Solid Edge part; units mm, degrees
sketch "Sketch1" plane through (0, 0, 0) normal (1, 0, 0) x (0, 1, 0)
  circle A0 centre (0, 0) radius 3.5
extrude "Protrusion1" add sketch "Sketch1" along normal mid plane 72
sketch "Sketch2" plane through (0, 0, 0) normal (0, -1, 0) x (1, 0, 0)
  line L0 (-36, 3) -> (-23, 3)
  line L1 (-23, 3) -> (-23, 3.5)
  dimension "D1" = 36
revolve "RevolvedCutout1" cut sketch "Sketch2" angle 360 about axis through (-60, 0, 0) along (1, 0, 0) material side at (-29.5, 0, 3.05)
sketch "Sketch3" plane through (0, 0, 0) normal (0, -1, 0) x (1, 0, 0)
  line L0 (36, 3) -> (2, 3)
  line L1 (2, 3) -> (2, 3.5)
  dimension "D1" = 36
revolve "RevolvedCutout2" cut sketch "Sketch3" angle 360 about axis through (-60, 0, 0) along (1, 0, 0) material side at (19, 0, 3.05)
sketch "Sketch4" plane through (0, 0, 0) normal (0, -1, 0) x (1, 0, 0)
  line L0 (16.5, 2.5) -> (16.5, 3)
  line L1 (21.5, 2.5) -> (16.5, 2.5)
  line L2 (21.5, 2.25) -> (21.5, 2.5)
  line L3 (21.5, 2.25) -> (26, 2.25)
  line L4 (26, 2.25) -> (26, 2)
  line L5 (26, 2) -> (36, 2)
  dimension "D1" = 26
revolve "RevolvedCutout3" cut sketch "Sketch4" angle 360 about axis through (-60, 0, 0) along (1, 0, 0) material side at (16.55, 0, 2.75)
cosmetic_thread "Gewinde_1" thread depth 9.5
fillet "Verrundung_2" radius 0.5 1 edges at (26, 0, -2)
sketch "Sketch5" plane through (0, 0, 0) normal (0, 0, 1) x (1, 0, 0)
  circle A0 centre (-19.75, 0) radius 1.25
extrude "Cutout1" cut sketch "Sketch5" along normal up to next and the other way up to next
sketch "Sketch6" plane through (0, 0, 0) normal (0, 0, 1) x (1, 0, 0)
  circle A0 centre (11.25, 0) radius 1.25
extrude "Cutout2" cut sketch "Sketch6" along normal up to next and the other way up to next
properties material "Stahl - Unlegierter:1.1191 , C45E"
Geometry check sheet. Reference: the model listing, model coordinates, mm. A direction names the side the tool comes from. Round coordinates to 2 decimals unless told otherwise and drop trailing zeros. Order: outer loops, then holes, each group sorted by start corner. A loop starts at its lowest first (then second) coordinate and runs counter-clockwise, first axis right, second up. Notation, with made-up numbers: (43, -23.75) - (76, -23.75) arc R35 ccw to (76, 8.25) - close; hole circle Ø6 at (19, -24.75). An arc over 180 degrees is marked (long way). Use a Markdown table: item, result. Add a question column.
(1) Sectioned sample at B-B, the plane z = 0. Enter the section's corners in (x, y).
(2) Release check for a two-part mould opening along X. For faces 1 (the flat face through (-36, 0, 0)), 2 (the cylindrical face through (-18.595, 0.479, -0.049)), 3 (the cylindrical face through (23.78, -2.23, -0.29)) record: pulls with the +X half, pulls with the -X half, needs draft (parallel to the pull), parting line crosses it, or undercut.
(3) Tool access check on faces 4 (the cylindrical face through (-10.675, 3.233, 1.341)), 5 (the flat face through (2, -1, 3)), 6 (the flat face through (-23, -1, 3)). Record the directions out of +Z, -Z, +X, -X, +Y, -Y that give a thin tool (end or side, any length) a straight path to the whole face; none if there is none.
(4) Sectioned sample at A-A, the plane y = 0. Count the separate pieces of the cut face and the enclosed holes in it, and give its area (3 significant figures).
(5) Depth check by flat-ended pin: pin 1 (1 mm diameter, centred on x = 10, y = -0.5, fed in from -Z); pin 2 (3 mm diameter, centred on x = -19.75, y = 0, fed in from -Z); pin 3 (1 mm diameter, centred on y = -2.5, z = -2.5, fed in from +X). Enter the tip coordinate at first touch or a pass-through.
(6) Sectioned sample at C-C, the plane x = 11.25. Enter the section's corners in (y, z).
(7) Sectioned sample at D-D, the plane x = -14. Enter the section's corners in (y, z), and give its area (3 significant figures).
(8) Material ranges on line 1 along X through (y, z) = (0, -0.25); line 2 along Y through (x, z) = (-19.75, 0.25); line 3 along X through (y, z) = (-0.75, -2), recorded low to high. Write a range as [from, to].
Answers below:
| question | item | result |
|---|---|---|
| 1 | outline | (-36, -3) - (-23, -3) - (-23, -3.5) - (2, -3.5) - (2, -3) - (16.5, -3) - (16.5, -2.5) - (21.5, -2.5) - (21.5, -2.25) - (26, -2.25) arc R0.5 cw to (26.43, -2) - (36, -2) - (36, 2) - (26.43, 2) arc R0.5 cw to (26, 2.25) - (21.5, 2.25) - (21.5, 2.5) - (16.5, 2.5) - (16.5, 3) - (2, 3) - (2, 3.5) - (-23, 3.5) - (-23, 3) - (-36, 3) - close; hole circle Ø2.5 at (-19.75, 0); hole circle Ø2.5 at (11.25, 0) |
| 2 | face 1 | pulls with the -X half |
| 2 | face 2 | undercut |
| 2 | face 3 | needs draft |
| 3 | face 4 | +X, -X |
| 3 | face 5 | +X |
| 3 | face 6 | -X |
| 4 | separate pieces | 3 |
| 4 | enclosed holes | 0 |
| 4 | area | 393 mm² |
| 5 | pin 1 | z = -3 |
| 5 | pin 2 | z = -3.5 |
| 5 | pin 3 | x = 2 |
| 6 | outline | (-1.25, -2.73) - (-1.25, 2.73) arc R3 ccw to start; (1.25, -2.73) arc R3 ccw to (1.25, 2.73) - close |
| 7 | outline | circle Ø7 at (0, 0) |
| 7 | area | 38.5 mm² |
| 8 | line 1 | [-36, -21], [-18.5, 10], [12.5, 36] |
| 8 | line 2 | [-3.49, -1.25], [1.25, 3.49] |
| 8 | line 3 | [-36, -20.75], [-18.75, 10.25], [12.25, 26.09] |
